Can you work these out from the model? Positions are in its coordinate system, mm. Face numbers are marked on the shaded views. A direction names the side the tool comes from. Coordinates: 2 decimals unless noted, no trailing zeros. Order: outer loops, then holes, each group sorted by start corner. A loop starts at its lowest first (then second) coordinate and runs counter-clockwise, first axis right, second up. Notation, with made-up numbers: (51, 82) -> (85, 82) arc R19 ccw to (85, 94) -> close; hole circle Ø11 at (78.25, 67). An arc over 180 degrees is marked (long way). Answer in a Markdown table with one row per item.
```python
from build123d import *

# Parameters (mm, degrees)
SKETCH1_R           = 2
SKETCH1_R_2         = 3
BOSS_EXTRUDE1_DEPTH = 5
SKETCH1_3_R         = 1.74625
BOSS_EXTRUDE2_DEPTH = 15
FILLET1_R           = 3


with BuildPart() as part:
    # Sketch1 → Boss-Extrude1 (new body)
    with BuildSketch(Plane.XY):
        with BuildLine():
            Line((10, -23.8), (10, -5.75))
            Line((10, -5.75), (-10, -5.75))
            Line((-10, -5.75), (-10, -23.8))
            ThreePointArc((-10, -23.8), (0, -33.8), (10, -23.8))
        make_face()
        with Locations((0, -23.8)):
            Circle(SKETCH1_R, mode=Mode.SUBTRACT)
        with Locations((0, -11.5)):
            Circle(SKETCH1_R_2, mode=Mode.SUBTRACT)
    extrude(amount=BOSS_EXTRUDE1_DEPTH)

    # Sketch1<3> → Boss-Extrude2 (add)
    with BuildSketch(Plane.XY):
        with BuildLine():
            Line((10, -5.75), (10, 0))
            ThreePointArc((10, 0), (0, 10), (-10, 0))
            Line((-10, 0), (-10, -5.75))
            Line((-10, -5.75), (10, -5.75))
        make_face()
        Circle(SKETCH1_3_R, mode=Mode.SUBTRACT)
    extrude(amount=BOSS_EXTRUDE2_DEPTH)

    # Fillet1
    fillet1_edges = [part.edges().sort_by_distance(p)[0] for p in [
        (-10, -5.75, 10),
        (10, -5.75, 10),
    ]]
    fillet(fillet1_edges, radius=FILLET1_R)


solid = part.part
```
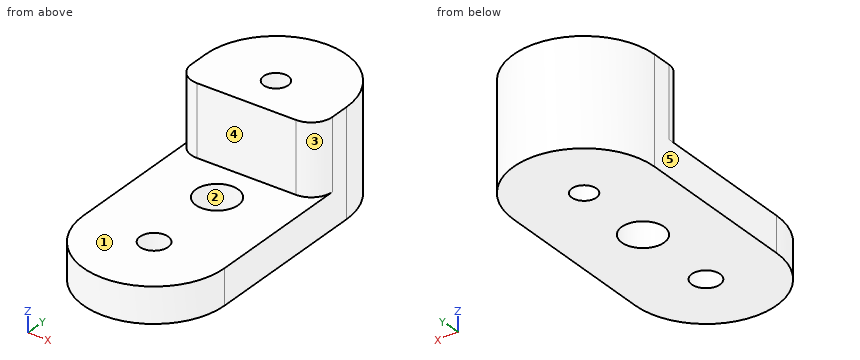
(1) Suppose I cut it at A-A (x = 0). Please give me the cut outline in (y, z).
Response values:
| item | result |
|---|---|
| outline | (-33.8, 0) -> (-25.8, 0) -> (-25.8, 5) -> (-33.8, 5) -> close; (-21.8, 0) -> (-14.5, 0) -> (-14.5, 5) -> (-21.8, 5) -> close; (-8.5, 0) -> (-1.75, 0) -> (-1.75, 15) -> (-5.75, 15) -> (-5.75, 5) -> (-8.5, 5) -> close; (1.75, 0) -> (10, 0) -> (10, 15) -> (1.75, 15) -> close |
(2) Will these pins go through, and if not, where does the flat tip stop? pin 1 Ø2 at (x, z) = (-4, 8) entering from -Y; pin 2 Ø3 at (y, z) = (-25.5, 5) entering from +X; pin 3 Ø3 at (x, z) = (-3, 7.5) entering from +Y.
Response values:
| item | result |
|---|---|
| pin 1 | y = -5.75 |
| pin 2 | x = 10 |
| pin 3 | y = 9.89 |
(3) I need wall thicknesses on line 1 (Y direction, x = 0, z = 1.7); line 2 (Z direction, x = 6, y = -9); line 3 (X direction, y = -23, z = 1.5). Which ranges of each line are inside material? Lowest first, please. Write a range as [from, to].
Response values:
| item | result |
|---|---|
| line 1 | [-33.8, -25.8], [-21.8, -14.5], [-8.5, -1.75], [1.75, 10] |
| line 2 | [0, 5] |
| line 3 | [-10, -1.83], [1.83, 10] |
(4) Suppose I cut it at B-B (y = -11.5). Please give me the cut outline in (x, z).
Response values:
| item | result |
|---|---|
| outline | (-10, 0) -> (-3, 0) -> (-3, 5) -> (-10, 5) -> close; (3, 0) -> (10, 0) -> (10, 5) -> (3, 5) -> close |
(5) On a 3-axis mill with a long thin cutter (end or side, diameter ignored), from which of +Z, -Z, +X, -X, +Y, -Y can I reach the whole of each face in a straight line? I mean the marked faces 4 and 5. Say none if no direction works.
Response values:
| item | result |
|---|---|
| face 4 | +Z, +X, -X, -Y |
| face 5 | +Z, -Z, -X, +Y, -Y |
(6) Suppose I cut it at C-C (z = 1). Please give me the cut outline in (x, y).
Response values:
| item | result |
|---|---|
| outline | (-10, -23.8) arc R10 ccw to (10, -23.8) -> (10, 0) arc R10 ccw to (-10, 0) -> close; hole circle Ø6 at (0, -11.5); hole circle Ø4 at (0, -23.8); hole circle Ø3.49 at (0, 0) |
(7) We'd pull the mould along X, two halves only. Please class the marked faces 1, 2 and 3: +X half, -X half, draft (parallel to the pull), parting line (faces both ways), or undercut.
Response values:
| item | result |
|---|---|
| face 1 | draft |
| face 2 | undercut |
| face 3 | +X half |
(8) Suppose I cut it at D-D (z = 5.5). Please give me the cut outline in (x, y).
Response values:
| item | result |
|---|---|
| outline | (-10, -2.75) arc R3 ccw to (-7, -5.75) -> (7, -5.75) arc R3 ccw to (10, -2.75) -> (10, 0) arc R10 ccw to (-10, 0) -> close; hole circle Ø3.49 at (0, 0) |
